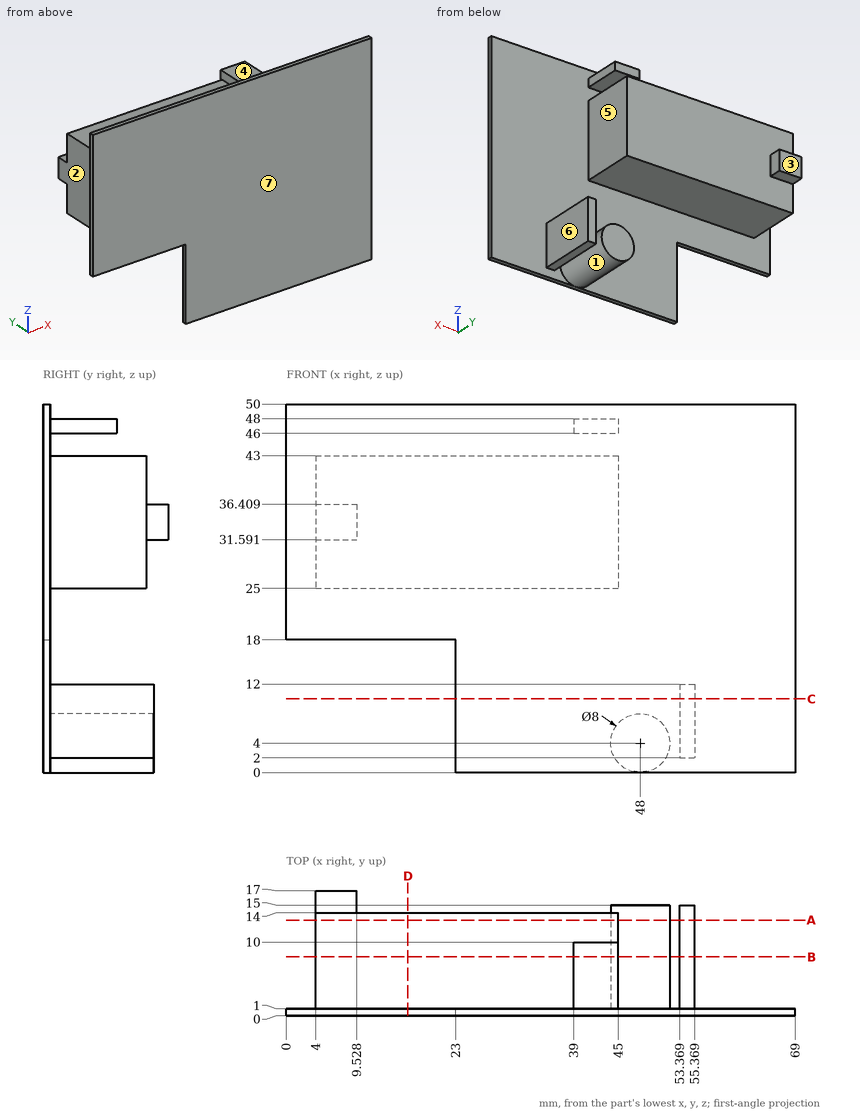
Source: three-view drawing plus pictorial views. Frame: mm from the lowest corner of the part. A direction names the side the tool comes from. Give positions to 0.01 mm unless a question says otherwise; leave off trailing zeros. Write each loop counter-clockwise with the first axis right and the second up, starting at its lowest first coordinate (ties: lowest second). Pieces come first, ordered by that corner, then holes. Notation, with made-up numbers: (27, 2) - (79, 2) arc R28 ccw to (79, 32) - close; hole circle Ø6 at (74.25, -25.75). An arc over 180 degrees is marked (long way). Write item = value, one per line. Start each with the question number.
Q1. Pin query (flat end, axial travel): pin 1 Ø8 at (y, z) = (12, 32.5) entering from -X; pin 2 Ø1 at (x, z) = (42, 47.5) entering from +Y; pin 3 Ø2.5 at (x, y) = (7, 15.5) entering from -Z. Return the tip coordinate at first contact, or that it passes through.
Q2. Reachability of the marked faces 4, 5, 6 and 7 from +Z, -Z, +X, -X, +Y, -Y: full face, straight path, thin tool, end or side. Return the list, or none.
Q3. Material intervals for probe 1 along Z at (x, y) = (40.5, 2); probe 2 along Y at (x, z) = (64, 32); probe 3 along Z at (x, y) = (6.5, 9.75), sorted ascending.
Q4. Cut plane D-D, the plane x = 16.5. Return loops of the section in (y, z).
Q5. Draft query along X for the marked faces 1, 2 and 3. Return one class per face: +X half, -X half, draft (parallel to the pull), parting line (faces both ways), or undercut.
Q6. Cut plane B-B, the plane y = 8. Return loops of the section in (x, z), then the cut area to 3 significant figures.
Q7. Cut plane A-A, the plane y = 13. Return loops of the section in (x, z).
Q8. Cut plane C-C, the plane z = 10. Return loops of the section in (x, y).
Computed values:
q1.pin_1 = 4
q1.pin_2 = 10
q1.pin_3 = 31.59
q2.face_4 = +Z, +X, -X, +Y
q2.face_5 = +Z, +X, +Y
q2.face_6 = +Z, -Z, +X, +Y
q2.face_7 = +Z, -Z, +X, -X, -Y
q3.probe_1 = 25 to 43, 46 to 48
q3.probe_2 = 0 to 1
q3.probe_3 = 25 to 43
q4.outline = (0, 18) - (1, 18) - (1, 25) - (14, 25) - (14, 43) - (1, 43) - (1, 50) - (0, 50) - close
q5.face_1 = undercut
q5.face_2 = -X half
q5.face_3 = draft
q6.outline = (4, 25) - (45, 25) - (45, 43) - (4, 43) - close; (39, 46) - (45, 46) - (45, 48) - (39, 48) - close; circle Ø8 at (48, 4); (53.37, 2) - (55.37, 2) - (55.37, 12) - (53.37, 12) - close
q6.area = 820 mm²
q7.outline = (4, 25) - (45, 25) - (45, 43) - (4, 43) - close; circle Ø8 at (48, 4); (53.37, 2) - (55.37, 2) - (55.37, 12) - (53.37, 12) - close
q8.outline = (23, 0) - (69, 0) - (69, 1) - (55.37, 1) - (55.37, 15) - (53.37, 15) - (53.37, 1) - (23, 1) - close
